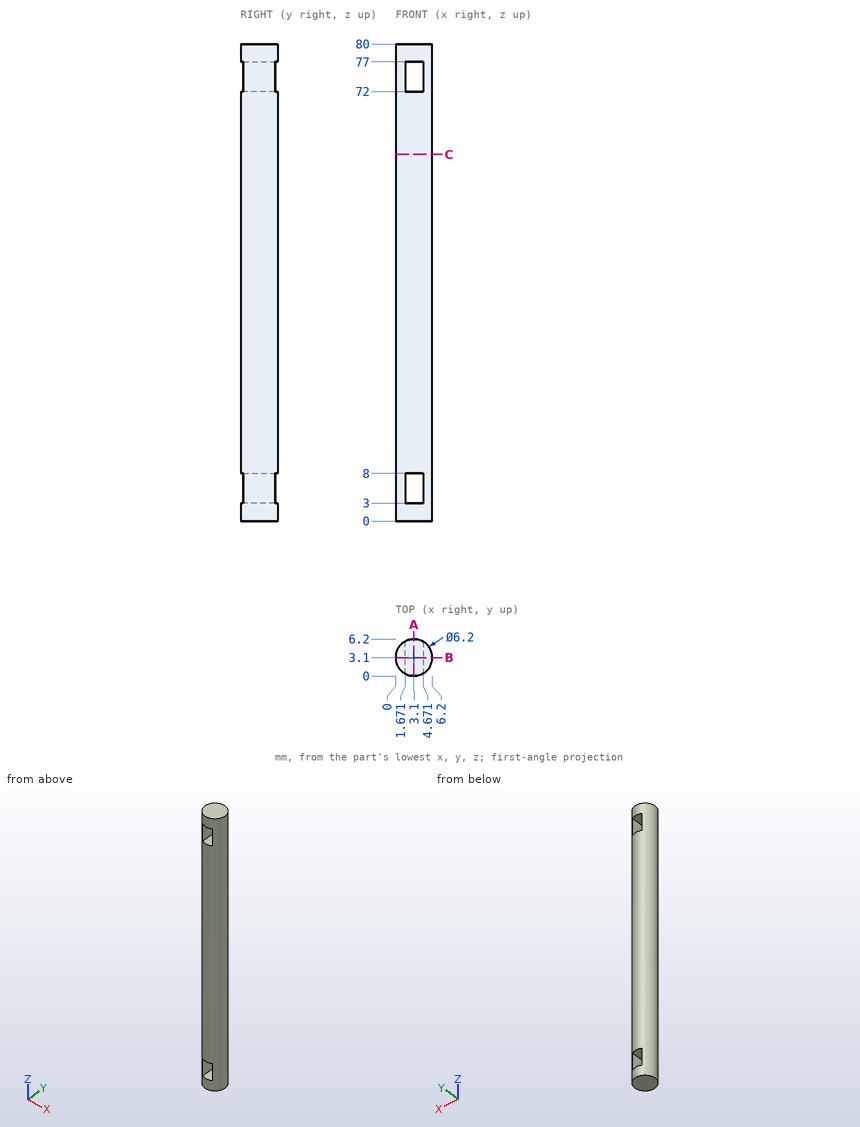
Geometry check sheet. Reference: drawing and pictorial views, mm from the part's lowest x, y, z. Coordinates: 2 decimals unless noted, no trailing zeros. Write each loop counter-clockwise with the first axis right and the second up, starting at its lowest first coordinate (ties: lowest second). Pieces come first, ordered by that corner, then holes. Notation, with made-up numbers: M -13.5,-32.5 L 40.5,-32.5 A10 ccw 40.5,-18.5 Z; hole C 61,11.25 d6. An arc over 180 degrees is marked long. Use one line per item in the form item = value.
Item 1: Gauge pin test, flat end, axial feed: pin 1 Ø1.5 at (y, z) = (4, 6) entering from -X. Record the tip position at first contact, or that the pin passes through.
Answer below:
pin_1 = 0
Item 2: Sectioned sample at A-A, the plane x = 3.1. Record the cut outline in (y, z), and give its area (3 significant figures).
Answer below:
outline = M 0,0 L 6.2,0 L 6.2,3 L 0,3 Z; M 0,8 L 6.2,8 L 6.2,72 L 0,72 Z; M 0,77 L 6.2,77 L 6.2,80 L 0,80 Z
area = 434 mm^2
Item 3: Sectioned sample at B-B, the plane y = 3.1. Record the cut outline in (x, z), and give its area (3 significant figures).
Answer below:
outline = M 0,0 L 6.2,0 L 6.2,80 L 0,80 Z; hole M 1.67,3 L 4.67,3 L 4.67,8 L 1.67,8 Z; hole M 1.67,72 L 4.67,72 L 4.67,77 L 1.67,77 Z
area = 466 mm^2
Item 4: Sectioned sample at C-C, the plane z = 61.5. Record the cut outline in (x, y), and give its area (3 significant figures).
Answer below:
outline = C 3.1,3.1 d6.2
area = 30.2 mm^2
Item 5: Material ranges on L1, parallel to Z at x = 1.75, y = 0.75; L2, parallel to Y at x = 4.5, z = 17 (1 decimal); L3, parallel to X at y = 1.25, z = 7.5, recorded low to high. Write a range as from..to.
Answer below:
L1 = 0..3, 8..72, 77..80
L2 = 0.3..5.9
L3 = 0.61..1.67, 4.67..5.59
